from build123d import *

# Parameters (mm, degrees)
BOSS_EXTRU_1_DEPTH       = 2
BOSS_EXTRU_1_DEPTH_BACK  = 5
ESQUISSE1_R              = 2
ESQUISSE1_R_2            = 1
BOSS_EXTRU_2_START       = 2
BOSS_EXTRU_2_OUTLINE_R   = 2
BOSS_EXTRU_2_DEPTH       = 2
BOSS_EXTRU_2_START_2     = 4
BOSS_EXTRU_2_2_OUTLINE_R = 2
BOSS_EXTRU_2_2_DEPTH     = 2
BOSS_EXTRU_2_START_3     = -3
BOSS_EXTRU_2_3_DEPTH     = 6
ENL_V_START              = -2
ESQUISSE4_R              = 1.5
ENL_V_MAT_EXTRU_1_DEPTH  = 2


with BuildPart() as part:
    # Esquisse1 → Boss.-Extru.1 (new, two sides: drawn at the far end of the back side and taken through both)
    with BuildSketch(Plane.XY.offset(-BOSS_EXTRU_1_DEPTH_BACK)):
        Circle(ESQUISSE1_R)
        Circle(ESQUISSE1_R_2, mode=Mode.SUBTRACT)
    extrude(amount=BOSS_EXTRU_1_DEPTH + BOSS_EXTRU_1_DEPTH_BACK)

    # Boss.-Extru.2: read off the stored shape, not the designer's step
    # Boss.-Extru.2 outline → Boss.-Extru.2 (add)
    with BuildSketch(Plane.XY.offset(BOSS_EXTRU_2_START)):
        Circle(BOSS_EXTRU_2_OUTLINE_R)
    extrude(amount=BOSS_EXTRU_2_DEPTH)

    # Boss.-Extru.2 2 outline → Boss.-Extru.2 2 (add)
    with BuildSketch(Plane.XY.offset(BOSS_EXTRU_2_START_2)):
        Circle(BOSS_EXTRU_2_2_OUTLINE_R)
    extrude(amount=BOSS_EXTRU_2_2_DEPTH)

    # Boss.-Extru.2 3 outline → Boss.-Extru.2 3 (cut)
    with BuildSketch(Plane(origin=(0, 0, 0), x_dir=(1, 0, 0), z_dir=(0, 1, 0)).offset(BOSS_EXTRU_2_START_3)):
        with BuildLine():
            Line((2, -3), (2, -4))
            ThreePointArc((2, -4), (1.414213562, -5.414213562), (0, -6))
            Line((0, -6), (3, -6))
            Line((3, -6), (3, -3))
            Line((3, -3), (2, -3))
        make_face()
        with BuildLine():
            Line((-3, -6), (0, -6))
            ThreePointArc((0, -6), (-1.414213562, -5.414213562), (-2, -4))
            Line((-2, -4), (-2, -3))
            Line((-2, -3), (-3, -3))
            Line((-3, -3), (-3, -6))
        make_face()
    extrude(amount=BOSS_EXTRU_2_3_DEPTH, mode=Mode.SUBTRACT)

    # Esquisse3 → Enlèvement de matière-Révolution1 (revolve, cut)
    with BuildSketch(Plane(origin=(0, 0, 0), x_dir=(0, 0, -1), z_dir=(1, 0, 0))):
        with BuildLine():
            Line((-4, -1), (-4, 1))
            ThreePointArc((-4, 1), (-3, 0), (-4, -1))
        make_face()
    revolve(axis=Axis((0, -1, 4), (0, 1, 0)), mode=Mode.SUBTRACT)

    # Esquisse4 → Enlèv. mat.-Extru.1 (cut)
    with BuildSketch(Plane(origin=(0, 2, 0), x_dir=(1, 0, 0), z_dir=(0, 1, 0)).offset(ENL_V_START)):
        with Locations(Location((0, -4, 0), (0, 0, 270))):
            Circle(ESQUISSE4_R)
    extrude(amount=ENL_V_MAT_EXTRU_1_DEPTH, mode=Mode.SUBTRACT)


solid = part.part
Geometry check sheet. Reference: the model listing, model coordinates, mm. A direction names the side the tool comes from. Round coordinates to 2 decimals unless told otherwise and drop trailing zeros. Order: outer loops, then holes, each group sorted by start corner. A loop starts at its lowest first (then second) coordinate and runs counter-clockwise, first axis right, second up. Notation, with made-up numbers: (18, 52.5) - (68, 52.5) arc R22 ccw to (68, 61.5) - close; hole circle Ø5 at (-39.5, 47). An arc over 180 degrees is marked (long way). One line per question, with ' | ' between items. Start each with the question number.
(1) Access from +Z, -Z, +X, -X, +Y, -Y to the whole of each face (thin tool, end or side, straight path). Record for faces 1 (the cylindrical face through (0, -1, -2)), 2 (the cylindrical face through (-0.575, 0.764, 5.386)).
(2) Sectioned sample at A-A on x = 1.2. Record the cut outline in (y, z), and give its area (3 significant figures).
(3) Sectioned sample at C-C on y = 0.4. Record the cut outline in (x, z).
(4) Depth check by flat-ended pin: pin 1 Ø2 at (x, y) = (0, 0.5) entering from -Z; pin 2 Ø1.5 at (x, z) = (0, 3.5) entering from +Y; pin 3 Ø1.5 at (x, y) = (-1, 0) entering from +Z; pin 4 Ø1.5 at (x, z) = (-1.5, 4.5) entering from -Y. Enter the tip coordinate at first touch or a pass-through.
(5) Sectioned sample at B-B on y = 1.75. Record the cut outline in (x, z).
(6) Sectioned sample at D-D on z = -2.5. Record the cut outline in (x, y), and give its area (3 significant figures).
(7) Release check for a two-part mould opening along Y. For faces 3 (the cylindrical face through (0.923, -1.774, 0.423)), 4 (the flat face through (0, 0, 2)), 5 (the flat face through (1, -1, -5)) record: released by +Y, released by -Y, zero draft, split by the parting line, or undercut.
(8) Thickness scan on L1, parallel to Y at x = 0, z = 0.25; L2, parallel to Z at x = 0.5, y = 0.4. Record the ranges inside material, lowest first. Write a range as [from, to].
Conclusion:
1) face 1: -Z | face 2: +Y
2) outline: (-1.6, -5) - (1.6, -5) - (1.6, 3.1) - (0, 3.1) - (0, 4.9) - (1.6, 4.9) - (1.6, 5.6) - (-1.6, 5.6) - close | area: 31.0 mm2
3) outline: (-1.96, -5) - (-0.92, -5) - (-0.92, 2) - (0.92, 2) - (0.92, -5) - (1.96, -5) - (1.96, 4.4) arc R2 ccw to (-1.96, 4.4) - close; hole circle Ø3 at (0, 4)
4) pin 1: stops at z = -5 | pin 2: stops at y = 0 | pin 3: stops at z = 5.98 | pin 4: stops at y = -1.85
5) outline: (-0.97, -5) - (0.97, -5) - (0.97, 2.85) arc R1.5 cw to (-0.97, 2.85) - close; (-0.97, 5.15) arc R1.5 cw to (0.97, 5.15) - (0.97, 5.75) arc R2 ccw to (-0.97, 5.75) - close
6) outline: circle Ø4 at (0, 0); hole circle Ø2 at (0, 0) | area: 9.42 mm2
7) face 3: split by the parting line | face 4: undercut | face 5: zero draft
8) L1: y = [-2, -1], [1, 2] | L2: z = [2, 2.59], [5.41, 5.94]
